Verification items for the finished model (mm, model axes). Face numbers are marked on the shaded views. A direction names the side the tool comes from. Give positions to 0.01 mm unless a question says otherwise; leave off trailing zeros. Loops run counter-clockwise (first coordinate to the right, second up) from the corner with the lowest first, then second, coordinate; pieces in that order, holes last. Notation, with made-up numbers: (-35, 29.5) - (-22, 29.5) arc R12 ccw to (-22, 42.5) - close; hole circle Ø8 at (11, -1). An arc over 180 degrees is marked (long way). Use one line per item in the form item = value.
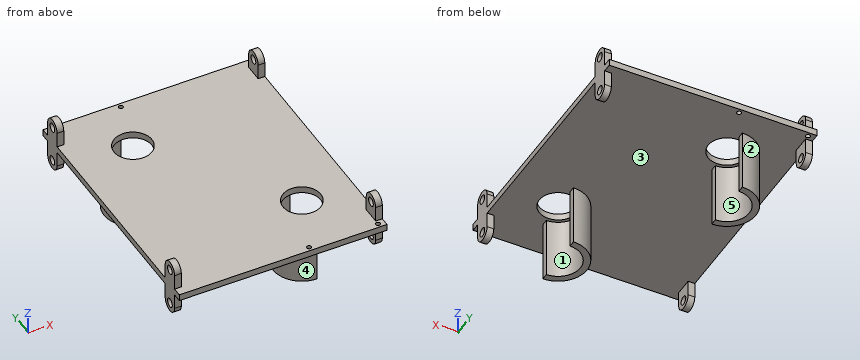
```python
from build123d import *

# Parameters (mm, degrees)
SKETCH1_W           = 93.5
SKETCH1_H           = 116
BOSS_EXTRUDE1_DEPTH = 3
SKETCH2_R           = 8.5
CUT_EXTRUDE1_DEPTH  = 75.555767718
SKETCH4_R           = 2
BOSS_EXTRUDE3_DEPTH = 3
SKETCH6_R           = 1
CUT_EXTRUDE2_DEPTH  = 10
BOSS_EXTRUDE4_DEPTH = 28


with BuildPart() as part:
    # Sketch1 → Boss-Extrude1 (new body)
    with BuildSketch(Plane.XY):
        Rectangle(SKETCH1_W, SKETCH1_H)
    extrude(amount=BOSS_EXTRUDE1_DEPTH)

    # Sketch2 → Cut-Extrude1 (cut, through all)
    with BuildSketch(Plane.XY.offset(3)):
        with Locations((-19.75, 32.5)):
            Circle(SKETCH2_R)
        with Locations((23.75, -29)):
            Circle(SKETCH2_R)
    extrude(amount=-CUT_EXTRUDE1_DEPTH, mode=Mode.SUBTRACT)

    # Sketch4 → Boss-Extrude3 (add)
    # profile 1 of 4: a face of its own
    with BuildSketch(Plane.ZY.offset(46.75)):
        with BuildLine():
            Line((-7, 54), (0, 54))
            Line((0, 54), (0, 46))
            Line((0, 46), (-7, 46))
            ThreePointArc((-7, 46), (-11, 50), (-7, 54))
        make_face()
        with Locations((-7, 50)):
            Circle(SKETCH4_R, mode=Mode.SUBTRACT)
    # profile 2 of 4: a face of its own
    with BuildSketch(Plane.ZY.offset(46.75)):
        with BuildLine():
            Line((0, -46), (-7, -46))
            ThreePointArc((-7, -46), (-11, -50), (-7, -54))
            Line((-7, -54), (0, -54))
            Line((0, -54), (0, -46))
        make_face()
        with Locations(Location((-7, -50, 0), (0, 0, 180))):
            Circle(SKETCH4_R, mode=Mode.SUBTRACT)
    # profile 3 of 4: a face of its own
    with BuildSketch(Plane.ZY.offset(46.75)):
        with BuildLine():
            Line((3, 46), (10, 46))
            ThreePointArc((10, 46), (14, 50), (10, 54))
            Line((10, 54), (3, 54))
            Line((3, 54), (3, 46))
        make_face()
        with Locations(Location((10, 50, 0), (0, 0, 180))):
            Circle(SKETCH4_R, mode=Mode.SUBTRACT)
    # profile 4 of 4: a face of its own
    with BuildSketch(Plane.ZY.offset(46.75)):
        with BuildLine():
            Line((10, -54), (3, -54))
            Line((3, -54), (3, -46))
            Line((3, -46), (10, -46))
            ThreePointArc((10, -46), (14, -50), (10, -54))
        make_face()
        with Locations((10, -50)):
            Circle(SKETCH4_R, mode=Mode.SUBTRACT)
    boss_extrude3 = extrude(amount=-BOSS_EXTRUDE3_DEPTH)

    # Sketch6 → Cut-Extrude2 (cut)
    with BuildSketch(Plane.XY.offset(3)):
        with Locations((-43.75, 56)):
            Circle(SKETCH6_R)
        with Locations((-12.75, 56)):
            Circle(SKETCH6_R)
        with Locations((43.75, -56)):
            Circle(SKETCH6_R)
        with Locations((12.75, -56)):
            Circle(SKETCH6_R)
    extrude(amount=-CUT_EXTRUDE2_DEPTH, mode=Mode.SUBTRACT)

    # Sketch5 → Boss-Extrude4 (add)
    with BuildSketch(Plane(origin=(0, 0, 0), x_dir=(-1, 0, 0), z_dir=(0, 0, -1))):
        with BuildLine():
            Line((19.75, 42.5), (19.75, 45.5))
            ThreePointArc((19.75, 45.5), (32.75, 32.5), (19.75, 19.5))
            Line((19.75, 19.5), (19.75, 22.5))
            ThreePointArc((19.75, 22.5), (29.75, 32.5), (19.75, 42.5))
        make_face()
        with BuildLine():
            Line((-23.75, -19), (-23.75, -16))
            ThreePointArc((-23.75, -16), (-10.75, -29), (-23.75, -42))
            Line((-23.75, -42), (-23.75, -39))
            ThreePointArc((-23.75, -39), (-13.75, -29), (-23.75, -19))
        make_face()
    extrude(amount=BOSS_EXTRUDE4_DEPTH)

    # Mirror1: Boss-Extrude3 across plane
    add(boss_extrude3.mirror(Plane(origin=(0, 0, 0), x_dir=(0, 0, 1), z_dir=(1, 0, 0))))


solid = part.part
```
1. Section check C-C, the plane y = 32.5. Record the cut outline in (x, z).
Result set:
outline = (-46.75, 0) - (-32.75, 0) - (-32.75, -28) - (-29.75, -28) - (-29.75, 0) - (-28.25, 0) - (-28.25, 3) - (-46.75, 3) - close; (-11.25, 0) - (46.75, 0) - (46.75, 3) - (-11.25, 3) - close
2. Section check A-A, the plane z = -24. Record the cut outline in (x, y), then the cut area to 3 significant figures.
Result set:
outline = (-19.75, 19.5) - (-19.75, 22.5) arc R10 cw to (-19.75, 42.5) - (-19.75, 45.5) arc R13 ccw to start; (23.75, -42) - (23.75, -39) arc R10 cw to (23.75, -19) - (23.75, -16) arc R13 ccw to start
area = 217 mm²
3. Depth check by flat-ended pin: pin 1 Ø1.5 at (x, y) = (22.5, -0.5) entering from -Z; pin 2 Ø0.9 at (x, z) = (-46, -2) entering from +Y; pin 3 Ø1.5 at (y, z) = (44, -13) entering from +X. Enter the tip coordinate at first touch or a pass-through.
Result set:
pin_1 = 0
pin_2 = 54
pin_3 = -19.75
4. Scan lines: probe 1 along Y at (x, z) = (-45, -7); probe 2 along Z at (x, y) = (25.5, 2.5); probe 3 along Y at (x, z) = (15.5, -17). Record each from-to range of solid material in increasing order.
Result set:
probe_1 = -54 to -52, -48 to -46, 46 to 48, 52 to 54
probe_2 = 0 to 3
probe_3 = -39.05 to -34.65, -23.35 to -18.95
5. Tool access check on the marked faces 3, 4 and 5. Record the directions out of +Z, -Z, +X, -X, +Y, -Y that give a thin tool (end or side, any length) a straight path to the whole face; none if there is none.
Result set:
face_3 = -Z
face_4 = -Z, -X
face_5 = -Z, +X
6. Section check D-D, the plane x = 28.5. Record the cut outline in (y, z).
Result set:
outline = (-58, 0) - (-36.05, 0) - (-36.05, 3) - (-58, 3) - close; (-21.95, 0) - (58, 0) - (58, 3) - (-21.95, 3) - close
7. Draft check along Y on the marked faces 1 and 2. Enter one of: released by +Y, released by -Y, zero draft, split by the parting line, or undercut.
Result set:
face_1 = undercut
face_2 = split by the parting line
8. Section check B-B, the plane z = -3. Record the cut outline in (x, y), then the cut area to 3 significant figures.
Result set:
outline = (-46.75, -54) - (-43.75, -54) - (-43.75, -46) - (-46.75, -46) - close; (-46.75, 46) - (-43.75, 46) - (-43.75, 54) - (-46.75, 54) - close; (-19.75, 19.5) - (-19.75, 22.5) arc R10 cw to (-19.75, 42.5) - (-19.75, 45.5) arc R13 ccw to start; (23.75, -42) - (23.75, -39) arc R10 cw to (23.75, -19) - (23.75, -16) arc R13 ccw to start; (43.75, -54) - (46.75, -54) - (46.75, -46) - (43.75, -46) - close; (43.75, 46) - (46.75, 46) - (46.75, 54) - (43.75, 54) - close
area = 313 mm²
